Verification items for the finished model (mm, model axes). Face numbers are marked on the shaded views. A direction names the side the tool comes from. Round coordinates to 2 decimals unless told otherwise and drop trailing zeros. Loops run counter-clockwise (first coordinate to the right, second up) from the corner with the lowest first, then second, coordinate; pieces in that order, holes last. Notation, with made-up numbers: (68.5, 66) -> (78.5, 66) arc R22 cw to (78.5, 93) -> close; hole circle Ø5 at (-30.75, 28). An arc over 180 degrees is marked (long way). Write item = value, one per line.
```python
from build123d import *

# Parameters (mm, degrees)
SKETCH1_W           = 24.13
SKETCH1_H           = 22.86
BOSS_EXTRUDE1_DEPTH = 3.175
SKETCH2_R           = 1.4732
CUT_EXTRUDE1_DEPTH  = 4.175
FILLET1_R           = 2.54
SKETCH3_W           = 6.35
SKETCH3_H           = 6.35
CUT_EXTRUDE2_DEPTH  = 4.175


with BuildPart() as part:
    # Sketch1 → Boss-Extrude1 (new body)
    with BuildSketch(Plane(origin=(0, 0, 0), x_dir=(1, 0, 0), z_dir=(0, 1, 0))):
        Rectangle(SKETCH1_W, SKETCH1_H)
    extrude(amount=BOSS_EXTRUDE1_DEPTH)

    # Sketch2 → Cut-Extrude1 (cut, through all)
    with BuildSketch(Plane(origin=(0, 3.175, 0), x_dir=(1, 0, 0), z_dir=(0, 1, 0))):
        with Locations((-6.985, 6.35)):
            Circle(SKETCH2_R)
        with Locations((-6.985, -6.35)):
            Circle(SKETCH2_R)
        with Locations((6.985, -6.35)):
            Circle(SKETCH2_R)
        with Locations((6.985, 6.35)):
            Circle(SKETCH2_R)
    extrude(amount=-CUT_EXTRUDE1_DEPTH, mode=Mode.SUBTRACT)

    # Fillet1
    fillet1_edges = [part.edges().sort_by_distance(p)[0] for p in [
        (12.065, 1.5875, 11.43),
        (-12.065, 1.5875, 11.43),
        (-12.065, 1.5875, -11.43),
        (12.065, 1.5875, -11.43),
    ]]
    fillet(fillet1_edges, radius=FILLET1_R)

    # Sketch3 → Cut-Extrude2 (cut, through all)
    with BuildSketch(Plane(origin=(0, 3.175, 0), x_dir=(1, 0, 0), z_dir=(0, 1, 0))):
        with Locations((0, 8.255)):
            Rectangle(SKETCH3_W, SKETCH3_H)
    extrude(amount=-CUT_EXTRUDE2_DEPTH, mode=Mode.SUBTRACT)


solid = part.part
```
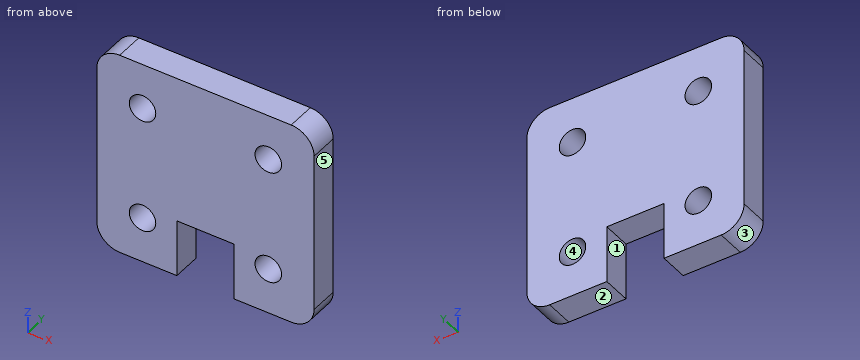
(1) Material ranges on probe 1 along X at (y, z) = (1.35, 6.35) (3 decimals); probe 2 along X at (y, z) = (1.65, -6.35) (3 decimals); probe 3 along Z at (x, y) = (-7, 2.4), recorded low to high. Write a range as from..to.
Filled sheet:
probe_1 = -12.065..-8.458, -5.512..5.512, 8.458..12.065
probe_2 = -12.065..-8.458, -5.512..-3.175, 3.175..5.512, 8.458..12.065
probe_3 = -11.43..-7.82, -4.88..4.88, 7.82..11.43
(2) Sectioned sample at C-C, the plane z = -5.5. Record the cut outline in (x, y) (3 decimals), and give its area (3 significant figures).
Filled sheet:
outline = (-12.065, 0) -> (-8.188, 0) -> (-8.188, 3.175) -> (-12.065, 3.175) -> close; (-5.782, 0) -> (-3.175, 0) -> (-3.175, 3.175) -> (-5.782, 3.175) -> close; (3.175, 0) -> (5.782, 0) -> (5.782, 3.175) -> (3.175, 3.175) -> close; (8.188, 0) -> (12.065, 0) -> (12.065, 3.175) -> (8.188, 3.175) -> close
area = 41.2 mm2
(3) Draft check along X on the marked faces 3, 4 and 5. Enter one of: released by +X, released by -X, zero draft, split by the parting line, or undercut.
Filled sheet:
face_3 = released by -X
face_4 = undercut
face_5 = released by +X
(4) Sectioned sample at B-B, the plane y = 1.05. Record the cut outline in (x, z) (3 decimals), and give its area (3 significant figures).
Filled sheet:
outline = (-12.065, -8.89) arc R2.54 ccw to (-9.525, -11.43) -> (-3.175, -11.43) -> (-3.175, -5.08) -> (3.175, -5.08) -> (3.175, -11.43) -> (9.525, -11.43) arc R2.54 ccw to (12.065, -8.89) -> (12.065, 8.89) arc R2.54 ccw to (9.525, 11.43) -> (-9.525, 11.43) arc R2.54 ccw to (-12.065, 8.89) -> close; hole circle Ø2.946 at (-6.985, -6.35); hole circle Ø2.946 at (-6.985, 6.35); hole circle Ø2.946 at (6.985, -6.35); hole circle Ø2.946 at (6.985, 6.35)
area = 478 mm2
(5) Sectioned sample at A-A, the plane z = 6.35. Record the cut outline in (x, y) (3 decimals).
Filled sheet:
outline = (-12.065, 0) -> (-8.458, 0) -> (-8.458, 3.175) -> (-12.065, 3.175) -> close; (-5.512, 0) -> (5.512, 0) -> (5.512, 3.175) -> (-5.512, 3.175) -> close; (8.458, 0) -> (12.065, 0) -> (12.065, 3.175) -> (8.458, 3.175) -> close
(6) Sectioned sample at D-D, the plane x = 0.5. Record the cut outline in (y, z) (3 decimals), and give its area (3 significant figures).
Filled sheet:
outline = (0, -5.08) -> (3.175, -5.08) -> (3.175, 11.43) -> (0, 11.43) -> close
area = 52.4 mm2
(7) Go/stop test with flat-tipped pins: pin 1 Ø2.5 at (x, z) = (-6.985, -6.35) entering from +Y; pin 2 Ø4.5 at (x, z) = (6.985, 6.35) entering from +Y (3 decimals). Record where each tip stops, or that it passes through.
Filled sheet:
pin_1 = through
pin_2 = 3.175
(8) Set-up check for the marked faces 1 and 2: record each of +Z, -Z, +X, -X, +Y, -Y from which the full face is reachable in a straight line by a thin tool's end or side.
Filled sheet:
face_1 = -Z, +Y, -Y
face_2 = -Z, +X, -X, +Y, -Y
